Build history of the part. All positions in model axes, mm. Give positions to 0.01 mm unless a question says otherwise; leave off trailing zeros. Loops run counter-clockwise (first coordinate to the right, second up) from the corner with the lowest first, then second, coordinate; pieces in that order, holes last. Notation, with made-up numbers: M -10,-14 L 45,-14 A18 ccw 45,18 Z; hole C 17,-33.75 d8. An arc over 180 degrees is marked long. Answer as a JSON object with one key per item and string values. Group by question number.
1. Slice it at C-C (z = 124.5). List the corners of the cut face in (x, y) (3 decimals), then the cut area to 3 significant figures.
2. Mould opens along Y. For faces 1 (the face through (-7.955, -6.1, 139.012)), 2 (the face through (9, -9, 0)), 3 (the face through (12.932, -5.362, 138.048)), 4 (the face through (-1.32, 10.06, 2.38)) say: released by +Y, released by -Y, zero draft, split by the parting line, or undercut.
3. Drill centre lines: line 1 along Y through (x, z) = (0, 139.5) (3 decimals); line 2 along X through (y, z) = (-8, 79); line 3 along X through (y, z) = (-4, 78.5). Where is each one in solid material? Low to high. Write a range as [from, to].
4. Drop flat-ended pins along their axis: pin 1 Ø2 at (y, z) = (6, 69) entering from -X; pin 2 Ø10 at (x, y) = (3, 6) entering from -Z; pin 3 Ø1.5 at (x, z) = (-6, 206.5) entering from -Y. Give the stop position or say it passes through.
5. Slice it at A-A (y = 0). List the corners of the cut face in (x, z) (3 decimals).
from build123d import *

# Parameters (mm, degrees)
F0_R     = 14
F0_R_2   = 10.025
F1_DEPTH = 280
F2_SIZE  = 0.6
F3_SIZE  = 2.5


with BuildPart() as f1:
    # F0 (on Top) → F1 (new body)
    with BuildSketch(Plane.XY):
        Circle(F0_R)
        Circle(F0_R_2, mode=Mode.SUBTRACT)
    extrude(amount=F1_DEPTH)

    # F2
    f2_edges = [f1.edges().sort_by_distance(p)[0] for p in [
        (-10.025, 0, 280),
        (-14, 0, 280),
        (-14, 0, 0),
    ]]
    chamfer(f2_edges, length=F2_SIZE)

    # F3
    f3_edges = [f1.edges().sort_by_distance(p)[0] for p in [
        (-10.025, 0, 0),
    ]]
    chamfer(f3_edges, length=F3_SIZE)


solid = f1.part
Established:
{
 "1": {"outline": "C 0,0 d28; hole C 0,0 d20.05", "area": "300 mm^2"},
 "2": {"face 1": "undercut", "face 2": "zero draft", "face 3": "split by the parting line", "face 4": "undercut"},
 "3": {"line 1": "y = [-14, -10.025], [10.025, 14]", "line 2": "x = [-11.49, -6.04], [6.04, 11.49]", "line 3": "x = [-13.42, -9.19], [9.19, 13.42]"},
 "4": {"pin 1": "stops at x = -13.08", "pin 2": "stops at z = 0.82", "pin 3": "stops at y = -12.98"},
 "5": {"outline": "M -14,0.6 L -13.4,0 L -12.525,0 L -10.025,2.5 L -10.025,279.4 L -10.625,280 L -13.4,280 L -14,279.4 Z; M 10.025,2.5 L 12.525,0 L 13.4,0 L 14,0.6 L 14,279.4 L 13.4,280 L 10.625,280 L 10.025,279.4 Z"}
}
